Design review of the part built by this model. Coordinates are the model's own, in mm. Face numbers are marked on the shaded views. A direction names the side the tool comes from. Coordinates: 2 decimals unless noted, no trailing zeros. Write each loop counter-clockwise with the first axis right and the second up, starting at its lowest first coordinate (ties: lowest second). Pieces come first, ordered by that corner, then holes. Notation, with made-up numbers: M 21,-30.75 L 49,-30.75 A28 cw 49,-4.75 Z; hole C 19.5,-33 d8. An arc over 180 degrees is marked long. Return JSON: item names as keys, results as strings. Group by question number.
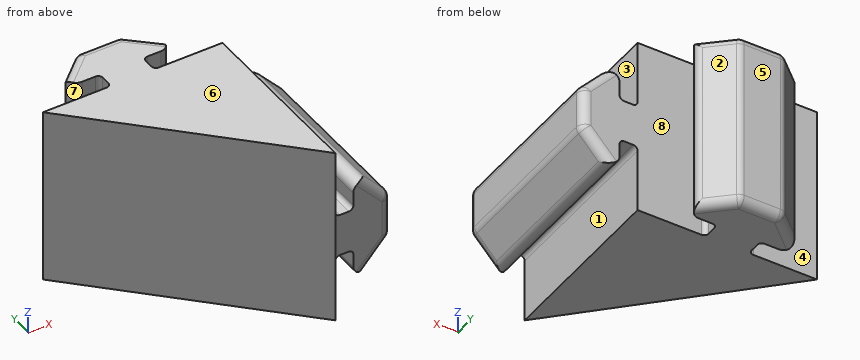
```python
from build123d import *

# Parameters (mm, degrees)
BOSS_EXTRUDE1_DEPTH = 20
BOSS_EXTRUDE2_DEPTH = 20
FILLET3_R           = 1
FILLET4_R           = 0.5


with BuildPart() as part:
    # Sketch1 → Boss-Extrude1 (new body)
    with BuildSketch(Plane.XY):
        Polygon((7.6, 26.2), (12.4, 26.2), (17, 22), (12.4, 22), (12.4, 20), (20, 20), (20, 0), (0, 0), (0, 20), (7.6, 20), (7.6, 22), (3, 22), align=None)
    extrude(amount=-BOSS_EXTRUDE1_DEPTH)

    # Sketch2 → Boss-Extrude2 (add)
    with BuildSketch(Plane(origin=(0, 0, 0), x_dir=(0, 0, -1), z_dir=(0, -1, 0))):
        Polygon((7.6, 26.2), (12.4, 26.2), (17, 22), (12.4, 22), (12.4, 20), (20, 20), (20, 0), (0, 0), (0, 20), (7.6, 20), (7.6, 22), (3, 22), align=None)
    extrude(amount=-BOSS_EXTRUDE2_DEPTH)

    # SurfaceCut1
    split(bisect_by=Plane(origin=(10, 10, 0), x_dir=(0.7071067811865476, -0.7071067811865475, 0), z_dir=(0.7071067811865475, 0.7071067811865476, 0)), keep=Keep.TOP)

    # Fillet3
    fillet3_edges = [part.edges().sort_by_distance(p)[0] for p in [
        (5.3, 24.1, -20),
        (5.3, 24.1, 0),
        (10, 26.2, 0),
        (14.7, 24.1, 0),
        (17, 22, -10),
        (3, 22, -10),
        (7.6, 26.2, -10),
        (12.4, 26.2, -10),
        (24.1, 20, -14.7),
        (26.2, 10, -12.4),
        (22, 10, -17),
        (14.7, 24.1, -20),
        (24.1, 20, -5.3),
        (22, 10, -3),
        (26.2, 20, -10),
        (26.2, 10, -7.6),
        (24.1, 0, -14.7),
        (26.2, 0, -10),
        (24.1, 0, -5.3),
        (10, 26.2, -20),
    ]]
    fillet(fillet3_edges, radius=FILLET3_R)

    # Fillet4
    fillet4_edges = [part.edges().sort_by_distance(p)[0] for p in [
        (12.4, 22, -10),
        (12.4, 20, -10),
        (7.6, 20, -10),
        (7.6, 22, -10),
        (22, 10, -12.4),
        (20, 10, -12.4),
        (20, 10, -7.6),
        (22, 10, -7.6),
    ]]
    fillet(fillet4_edges, radius=FILLET4_R)


solid = part.part
```
Item 1: Add section C-C (z = -17.25). Write out the cut boundary in (x, y), plus the area to 3 significant figures.
Item 2: For line 1 (Y direction, x = 22.75, z = -6.25); line 2 (X direction, y = 12.25, z = -7.5); line 3 (X direction, y = 14.25, z = -7.25), list the stretches that pass through material, from the lowest coordinate up.
Item 3: Machinability: for the marked faces 1, 2, 3 and 4, which of the approach directions +Z, -Z, +X, -X, +Y, -Y give a long, thin tool a straight path to every point of the face, cutting with its end or side? Answer none if there is none.
Item 4: Add section A-A (x = 10.75). Write out the cut boundary in (y, z), plus the area to 3 significant figures.
Item 5: Add section D-D (y = 10). Write out the cut boundary in (x, z), plus the area to 3 significant figures.
Item 6: Add section B-B (y = 13.5). Write out the cut boundary in (x, z).
Item 7: For pin 1 (0.8 mm diameter, centred on y = 8, z = -6.5, fed in from -X); pin 2 (1.2 mm diameter, centred on x = 14, z = -8.5, fed in from -Y); pin 3 (6 mm diameter, centred on y = 21.5, z = -18, fed in from -X); pin 4 (0.8 mm diameter, centred on y = 21, z = -12.5, fed in from -X), all flat-tipped, find the tip position at first contact; note any pin that passes through.
Item 8: The part is to be moulded in two halves that separate along Y. For the marked faces 5, 6, 7 and 8, say which applies: pulls with the +Y half, pulls with the -Y half, needs draft (parallel to the pull), parting line crosses it, or undercut.
Geometry check:
{
 "1": {"outline": "M 0,20 L 20,0 L 20,20 L 12.9,20 A0.5 cw 12.4,20.5 L 12.4,21.5 A0.5 cw 12.9,22 L 14.42,22 A1 ccw 15.1,23.74 L 12.69,25.94 A1 ccw 12.01,26.2 L 7.99,26.2 A1 ccw 7.31,25.94 L 4.9,23.74 A1 ccw 5.58,22 L 7.1,22 A0.5 cw 7.6,21.5 L 7.6,20.5 A0.5 cw 7.1,20 Z", "area": "247 mm^2"},
 "2": {"line 1": "0 to 20", "line 2": "7.75 to 20.2, 21.8 to 26.07", "line 3": "5.75 to 20.02, 21.98 to 25.88"},
 "3": {"face 1": "-Z, +Y, -Y", "face 2": "+Z, -Z, +X, +Y", "face 3": "+Z, +Y, -Y", "face 4": "+Z, -Z, -X"},
 "4": {"outline": "M 9.25,-20 L 25.2,-20 A1 ccw 26.2,-19 L 26.2,-1 A1 ccw 25.2,0 L 9.25,0 Z", "area": "339 mm^2"},
 "5": {"outline": "M 10,-20 L 20,-20 L 20,-12.9 A0.5 cw 20.5,-12.4 L 21.5,-12.4 A0.5 cw 22,-12.9 L 22,-14.42 A1 ccw 23.74,-15.1 L 25.94,-12.69 A1 ccw 26.2,-12.01 L 26.2,-7.99 A1 ccw 25.94,-7.31 L 23.74,-4.9 A1 ccw 22,-5.58 L 22,-7.1 A0.5 cw 21.5,-7.6 L 20.5,-7.6 A0.5 cw 20,-7.1 L 20,0 L 10,0 Z", "area": "247 mm^2"},
 "6": {"outline": "M 6.5,-20 L 20,-20 L 20,-12.9 A0.5 cw 20.5,-12.4 L 21.5,-12.4 A0.5 cw 22,-12.9 L 22,-14.42 A1 ccw 23.74,-15.1 L 25.94,-12.69 A1 ccw 26.2,-12.01 L 26.2,-7.99 A1 ccw 25.94,-7.31 L 23.74,-4.9 A1 ccw 22,-5.58 L 22,-7.1 A0.5 cw 21.5,-7.6 L 20.5,-7.6 A0.5 cw 20,-7.1 L 20,0 L 6.5,0 Z"},
 "7": {"pin 1": "x = 11.6", "pin 2": "y = 5.4", "pin 3": "x = 0", "pin 4": "x = 7.6"},
 "8": {"face 5": "pulls with the +Y half", "face 6": "needs draft", "face 7": "undercut", "face 8": "undercut"}
}
